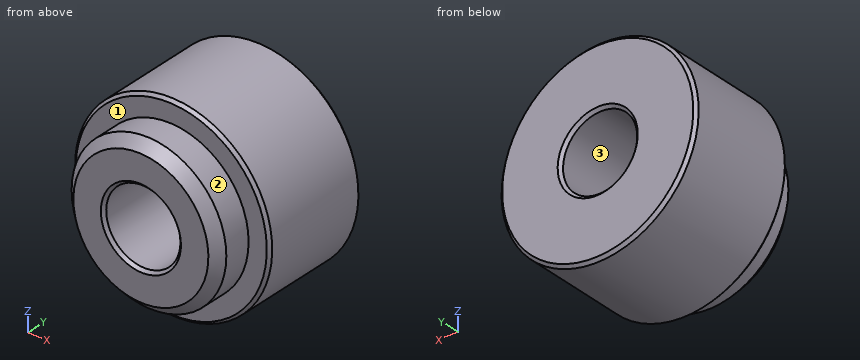
from build123d import *

# Parameters (mm, degrees)
F2_SIZE = 2.54
F3_SIZE = 0.762


with BuildPart() as f1:
    # F0 (on Right) → F1 (revolve)
    with BuildSketch(Plane.YZ):
        Polygon((9.525, 19.939), (0, 19.939), (0, 9.5631), (38.1, 9.5631), (38.1, 25.4), (9.525, 25.4), align=None)
    revolve(axis=Axis((0, 8.629879, 0), (0, 1, 0)))

    # F2
    f2_edges = [f1.edges().sort_by_distance(p)[0] for p in [
        (0, 0, -19.939),
    ]]
    chamfer(f2_edges, length=F2_SIZE)

    # F3
    f3_edges = [f1.edges().sort_by_distance(p)[0] for p in [
        (0, 0, -9.5631),
        (0, 38.1, -9.5631),
        (0, 19.05, 9.5631),
        (0, 38.1, -25.4),
        (0, 9.525, -25.4),
        (0, 23.8125, 25.4),
    ]]
    chamfer(f3_edges, length=F3_SIZE)


solid = f1.part
The listing builds one solid part. Answer for the finished solid, in the listing's coordinates (mm). Face numbers are marked on the shaded views. Coordinates: 2 decimals unless noted, no trailing zeros. Loops run counter-clockwise (first coordinate to the right, second up) from the corner with the lowest first, then second, coordinate; pieces in that order, holes last. Notation, with made-up numbers: (43.5, 17) -> (79.5, 17) arc R15 ccw to (79.5, 29) -> close; hole circle Ø2 at (32, 19). An arc over 180 degrees is marked (long way). Write item = value, one per line. Start each with the question number.
1) Given pin 1 Ø10 at (x, z) = (-13.5, -13.5) entering from -Y; pin 2 Ø12 at (y, z) = (18, 18) entering from +X; pin 3 Ø10 at (x, y) = (10.5, 9.5) entering from -Z; pin 4 Ø2 at (y, z) = (25.5, 2.5) entering from -X, each flat-ended and moving along its own axis, determine where each tip first touches the part or whether it passes through.
2) A cutting plane is placed at A-A (x = 0). Give the vertices of the cut face in (y, z) (3 decimals), then the cut area to 3 significant figures.
3) The mould has two halves that part along X. Classify the marked faces 1, 2 and 3: released by +X, released by -X, zero draft, split by the parting line, or undercut.
4) Straight lines are drawn through the part: line 1 (X direction, y = 19, z = 0); line 2 (Y direction, x = -4, z = -22.5) (3 decimals); line 3 (X direction, y = 10, z = 0). For each, find the intervals that lie inside material, in ascending order. Write a range as from..to.
5) A cutting plane is placed at C-C (y = 12). Give the vertices of the cut face in (x, z), then the cut area to 3 significant figures.
6) A cutting plane is placed at B-B (z = 0). Give the vertices of the cut face in (x, y) (3 decimals).
Responses:
q1.pin_1 = 0
q1.pin_2 = 22.39
q1.pin_3 = -24.78
q1.pin_4 = -25.36
q2.outline = (0, -17.399) -> (2.54, -19.939) -> (9.525, -19.939) -> (9.525, -24.638) -> (10.287, -25.4) -> (37.338, -25.4) -> (38.1, -24.638) -> (38.1, -10.325) -> (37.338, -9.563) -> (0.762, -9.563) -> (0, -10.325) -> close; (0, 10.325) -> (0.762, 9.563) -> (37.338, 9.563) -> (38.1, 10.325) -> (38.1, 24.638) -> (37.338, 25.4) -> (10.287, 25.4) -> (9.525, 24.638) -> (9.525, 19.939) -> (2.54, 19.939) -> (0, 17.399) -> close
q2.area = 1,090 mm²
q3.face_1 = zero draft
q3.face_2 = split by the parting line
q3.face_3 = undercut
q4.line_1 = -25.4..-9.56, 9.56..25.4
q4.line_2 = 9.525..38.1
q4.line_3 = -25.11..-9.56, 9.56..25.11
q5.outline = circle Ø50.8 at (0, 0); hole circle Ø19.13 at (0, 0)
q5.area = 1,740 mm²
q6.outline = (-25.4, 10.287) -> (-24.638, 9.525) -> (-19.939, 9.525) -> (-19.939, 2.54) -> (-17.399, 0) -> (-10.325, 0) -> (-9.563, 0.762) -> (-9.563, 37.338) -> (-10.325, 38.1) -> (-24.638, 38.1) -> (-25.4, 37.338) -> close; (9.563, 0.762) -> (10.325, 0) -> (17.399, 0) -> (19.939, 2.54) -> (19.939, 9.525) -> (24.638, 9.525) -> (25.4, 10.287) -> (25.4, 37.338) -> (24.638, 38.1) -> (10.325, 38.1) -> (9.563, 37.338) -> close
